```python
from build123d import *

# Parameters (mm, degrees)
BOSS_EXTRU_3_DEPTH = 2
BOSS_EXTRU_4_DEPTH = 10


with BuildPart() as part:
    # Esquisse1 → Boss.-Extru.3 (new body)
    with BuildSketch(Plane.XY):
        with BuildLine():
            Line((-70, 0), (-10.000000065, 0))
            ThreePointArc((-10.000000065, 0), (-2.928932211, 2.928932165), (0, 10))
            Line((0, 10), (0, 110))
            ThreePointArc((0, 110), (-2.928932188, 117.071067812), (-10, 120))
            Line((-10, 120), (-70, 120))
            ThreePointArc((-70, 120), (-77.071067812, 117.071067812), (-80, 110))
            Line((-80, 110), (-80, 10))
            ThreePointArc((-80, 10), (-77.071067812, 2.928932188), (-70, 0))
        make_face()
    extrude(amount=BOSS_EXTRU_3_DEPTH)

    # Esquisse3 → Boss.-Extru.4 (add)
    with BuildSketch(Plane.XY.offset(2)):
        with BuildLine():
            ThreePointArc((-80, 10), (-79.486832981, 6.83772234), (-78, 4))
            Line((-78, 4), (-78, 10))
            Line((-78, 10), (-78, 16))
            ThreePointArc((-78, 16), (-79.486832981, 13.16227766), (-80, 10))
        make_face()
        with BuildLine():
            ThreePointArc((-78, 4), (-77.071067812, 2.928932188), (-76, 2))
            Line((-76, 2), (-70, 2))
            ThreePointArc((-70, 2), (-75.656854249, 4.343145751), (-78, 10))
            Line((-78, 10), (-78, 4))
        make_face()
        with BuildLine():
            ThreePointArc((-76, 2), (-73.16227766, 0.513167019), (-70, 0))
            ThreePointArc((-70, 0), (-66.83772234, 0.513167019), (-64, 2))
            Line((-64, 2), (-70, 2))
            Line((-70, 2), (-76, 2))
        make_face()
        with BuildLine():
            Line((-70, 0), (-10, 0))
            ThreePointArc((-10, 0), (-13.16227766, 0.513167019), (-16, 2))
            Line((-16, 2), (-64, 2))
            ThreePointArc((-64, 2), (-66.83772234, 0.513167019), (-70, 0))
        make_face()
        with BuildLine():
            ThreePointArc((-80, 10), (-79.486832981, 13.16227766), (-78, 16))
            Line((-78, 16), (-78, 104))
            ThreePointArc((-78, 104), (-79.486832981, 106.83772234), (-80, 110))
            Line((-80, 110), (-80, 10))
        make_face()
        with BuildLine():
            ThreePointArc((-80, 110), (-79.486832981, 106.83772234), (-78, 104))
            Line((-78, 104), (-78, 110))
            Line((-78, 110), (-78, 116))
            ThreePointArc((-78, 116), (-79.486832981, 113.16227766), (-80, 110))
        make_face()
        with BuildLine():
            ThreePointArc((-78, 110), (-75.656854249, 115.656854249), (-70, 118))
            Line((-70, 118), (-76, 118))
            ThreePointArc((-76, 118), (-77.071067812, 117.071067812), (-78, 116))
            Line((-78, 116), (-78, 110))
        make_face()
        with BuildLine():
            Line((-70, 118), (-64, 118))
            ThreePointArc((-64, 118), (-66.83772234, 119.486832981), (-70, 120))
            ThreePointArc((-70, 120), (-73.16227766, 119.486832981), (-76, 118))
            Line((-76, 118), (-70, 118))
        make_face()
        with BuildLine():
            Line((-64, 118), (-16, 118))
            ThreePointArc((-16, 118), (-13.16227766, 119.486832981), (-10, 120))
            Line((-10, 120), (-70, 120))
            ThreePointArc((-70, 120), (-66.83772234, 119.486832981), (-64, 118))
        make_face()
        with BuildLine():
            ThreePointArc((-10, 120), (-13.16227766, 119.486832981), (-16, 118))
            Line((-16, 118), (-10, 118))
            Line((-10, 118), (-4, 118))
            ThreePointArc((-4, 118), (-6.83772234, 119.486832981), (-10, 120))
        make_face()
        with BuildLine():
            Line((-2, 110), (-2, 116))
            ThreePointArc((-2, 116), (-2.928932188, 117.071067812), (-4, 118))
            Line((-4, 118), (-10, 118))
            ThreePointArc((-10, 118), (-4.343145751, 115.656854249), (-2, 110))
        make_face()
        with BuildLine():
            ThreePointArc((-2, 104), (-0.513167019, 106.83772234), (0, 110))
            ThreePointArc((0, 110), (-0.513167019, 113.16227766), (-2, 116))
            Line((-2, 116), (-2, 110))
            Line((-2, 110), (-2, 104))
        make_face()
        with BuildLine():
            ThreePointArc((-2, 16), (-0.513167019, 13.16227766), (0, 10))
            Line((0, 10), (0, 110))
            ThreePointArc((0, 110), (-0.513167019, 106.83772234), (-2, 104))
            Line((-2, 104), (-2, 16))
        make_face()
        with BuildLine():
            Line((-2, 10), (-2, 4))
            ThreePointArc((-2, 4), (-0.513167019, 6.83772234), (0, 10))
            ThreePointArc((0, 10), (-0.513167019, 13.16227766), (-2, 16))
            Line((-2, 16), (-2, 10))
        make_face()
        with BuildLine():
            Line((-10, 2), (-4, 2))
            ThreePointArc((-4, 2), (-2.928932188, 2.928932188), (-2, 4))
            Line((-2, 4), (-2, 10))
            ThreePointArc((-2, 10), (-4.343145751, 4.343145751), (-10, 2))
        make_face()
        with BuildLine():
            ThreePointArc((-10, 0), (-6.83772234, 0.513167019), (-4, 2))
            Line((-4, 2), (-10, 2))
            Line((-10, 2), (-16, 2))
            ThreePointArc((-16, 2), (-13.16227766, 0.513167019), (-10, 0))
        make_face()
    extrude(amount=BOSS_EXTRU_4_DEPTH)


solid = part.part
```
Here's how the part is built. I have some questions about the finished solid (model axes, mm). A direction names the side the tool comes from. Coordinates: 2 decimals unless noted, no trailing zeros. Write each loop counter-clockwise with the first axis right and the second up, starting at its lowest first coordinate (ties: lowest second). Pieces come first, ordered by that corner, then holes. Notation, with made-up numbers: (19, 9) -> (77, 9) arc R19 cw to (77, 16) -> close; hole circle Ø6 at (10, 67.25). An arc over 180 degrees is marked (long way). Use a Markdown table: item, result. Add a question column.
(1) If we section it at D-D, the plane y = 7: Write out the boundary of the cut face in (x, z), and give its area (3 significant figures).
(2) I'm going to push flat-ended pins straight in: P1, Ø10, axis at x = -33, y = 78.5, coming from the +Z side; P2, Ø8, axis at x = -59.5, y = 106.5, coming from the -Z side. Where does each tip first touch, or does it pass through?
(3) If we section it at C-C, the plane y = 25: Write out the boundary of the cut face in (x, z).
(4) We'd pull the mould along Y, two halves only. Please class faces 1 (the flat face through (-78, 59, 7)), 2 (the flat face through (-40, 120, 6)), 3 (the cylindrical face through (-75.594, 4.281, 6.93)), 4 (the flat face through (-40, 0, 6)): +Y half, -Y half, draft (parallel to the pull), parting line (faces both ways), or undercut.
(5) Please list where these lines run through material, in increasing order: line 1 (Y direction, x = -26.5, z = 5.75); line 2 (X direction, y = 63.5, z = 8); line 3 (Z direction, x = -13, y = 40).
(6) If we section it at A-A, the plane z = 7.25: Write out the boundary of the cut face in (x, y), and give its area (3 significant figures).
(7) For faces 5 (the cylindrical face through (-4.281, 4.406, 6.93)), 6 (the flat face through (-41, 61, 0)), which set-ups out of +Z, -Z, +X, -X, +Y, -Y let a thin tool reach every point of the face, with its end or its side?
(8) If we section it at B-B, the plane x = -61.5: Write out the boundary of the cut face in (y, z).
Outcome:
| question | item | result |
|---|---|---|
| 1 | outline | (-79.54, 0) -> (-0.46, 0) -> (-0.46, 12) -> (-2.58, 12) -> (-2.58, 2) -> (-77.42, 2) -> (-77.42, 12) -> (-79.54, 12) -> close |
| 1 | area | 201 mm^2 |
| 2 | P1 | stops at z = 2 |
| 2 | P2 | stops at z = 0 |
| 3 | outline | (-80, 0) -> (0, 0) -> (0, 12) -> (-2, 12) -> (-2, 2) -> (-78, 2) -> (-78, 12) -> (-80, 12) -> close |
| 4 | face 1 | undercut |
| 4 | face 2 | +Y half |
| 4 | face 3 | undercut |
| 4 | face 4 | -Y half |
| 5 | line 1 | y = 0 to 2, 118 to 120 |
| 5 | line 2 | x = -80 to -78, -2 to 0 |
| 5 | line 3 | z = 0 to 2 |
| 6 | outline | (-80, 10) arc R10 ccw to (-70, 0) -> (-10, 0) arc R10 ccw to (0, 10) -> (0, 110) arc R10 ccw to (-10, 120) -> (-70, 120) arc R10 ccw to (-80, 110) -> close; hole (-78, 10) arc R8 ccw to (-70, 2) -> (-10, 2) arc R8 ccw to (-2, 10) -> (-2, 110) arc R8 ccw to (-10, 118) -> (-70, 118) arc R8 ccw to (-78, 110) -> close |
| 6 | area | 753 mm^2 |
| 7 | face 5 | +Z |
| 7 | face 6 | -Z, +X, -X, +Y, -Y |
| 8 | outline | (0, 0) -> (120, 0) -> (120, 12) -> (118, 12) -> (118, 2) -> (2, 2) -> (2, 12) -> (0, 12) -> close |
